Could you check a few things on this model? Use its own coordinates, in mm. A direction names the side the tool comes from. Give positions to 0.01 mm unless a question says otherwise; leave off trailing zeros. Loops run counter-clockwise (first coordinate to the right, second up) from the corner with the lowest first, then second, coordinate; pieces in that order, holes last. Notation, with made-up numbers: M 19,61 L 44,61 A10 ccw 44,80 Z; hole C -9.75,30 d8. An arc over 180 degrees is marked long. Answer in a Markdown table with one row per item. Add a question column.
```python
from build123d import *

# Parameters (mm, degrees)
F0_W     = 13
F0_H     = 7
F1_DEPTH = 9
F2_R     = 1.5
F3_DEPTH = 9
F4_R     = 1
F5_DEPTH = 10


with BuildPart() as f1:
    # F0 (on Top) → F1 (new body)
    with BuildSketch(Plane.XY):
        Rectangle(F0_W, F0_H)
    extrude(amount=F1_DEPTH)

    # F2 (on face) → F3 (join)
    with BuildSketch(Plane.XY.offset(9)):
        Circle(F2_R)
    extrude(amount=F3_DEPTH)

    # F4 (on face) → F5 (join)
    with BuildSketch(Plane.XY.offset(18)):
        Circle(F4_R)
    extrude(amount=F5_DEPTH)


solid = f1.part
```
Item 1: For P1, Ø4, axis at x = -0.5, z = 24.5, coming from the +Y side, with a flat end and sliding along its axis, tell me the tip position at first contact or that it passes through.
Item 2: Suppose I cut it at D-D (y = 2.25). List the corners of the cut face in (x, z) for me.
Item 3: Suppose I cut it at A-A (y = 0). List the corners of the cut face in (x, z) for me.
Item 4: For faces 1 (the face through (0, -1, 23)), 2 (the face through (6.5, 0, 4)), which set-ups out of +Z, -Z, +X, -X, +Y, -Y let a thin tool reach every point of the face, with its end or its side?
Item 5: Suppose I cut it at B-B (x = 0). List the corners of the cut face in (y, z) for me, then the cut area to 3 significant figures.
Item 6: I need wall thicknesses on L1, parallel to Z at x = -1.25, y = 2.25; L2, parallel to Z at x = 0.5, y = 1.25; L3, parallel to Y at x = -0.25, z = 26. Which ranges of each line are inside material? Lowest first, please.
Item 7: Suppose I cut it at C-C (z = 17). List the corners of the cut face in (x, y) for me, then the cut area to 3 significant figures.
Values found:
| question | item | result |
|---|---|---|
| 1 | P1 | y = 1 |
| 2 | outline | M -6.5,0 L 6.5,0 L 6.5,9 L -6.5,9 Z |
| 3 | outline | M -6.5,0 L 6.5,0 L 6.5,9 L 1.5,9 L 1.5,18 L 1,18 L 1,28 L -1,28 L -1,18 L -1.5,18 L -1.5,9 L -6.5,9 Z |
| 4 | face 1 | +Z |
| 4 | face 2 | +Z, -Z, +X, +Y, -Y |
| 5 | outline | M -3.5,0 L 3.5,0 L 3.5,9 L 1.5,9 L 1.5,18 L 1,18 L 1,28 L -1,28 L -1,18 L -1.5,18 L -1.5,9 L -3.5,9 Z |
| 5 | area | 110 mm² |
| 6 | L1 | 0 to 9 |
| 6 | L2 | 0 to 18 |
| 6 | L3 | -0.97 to 0.97 |
| 7 | outline | C 0,0 d3 |
| 7 | area | 7.07 mm² |
